Part model, mm, in its own coordinate system. A direction names the side the tool comes from. Coordinates: 2 decimals unless noted, no trailing zeros. Loops run counter-clockwise (first coordinate to the right, second up) from the corner with the lowest first, then second, coordinate; pieces in that order, holes last. Notation, with made-up numbers: (-32.75, -22) - (10.25, -22) arc R23 cw to (10.25, -14) - close; hole circle Ø5 at (14.5, -35). An arc over 180 degrees is marked (long way). Answer as CSV lines item,"result".
Autodesk Inventor part; units mm, degrees
ref_plane "YZ Plane" through (0, 0, 0) normal (1, 0, 0) x (0, 1, 0)
ref_plane "XZ Plane" through (0, 0, 0) normal (0, 1, 0) x (-1, 0, 0)
ref_plane "XY Plane" through (0, 0, 0) normal (0, 0, 1) x (1, 0, 0)
sketch "Sketch1" plane through (0, 0, 0) normal (0, 0, 1) x (1, 0, 0)
  line L0 (-4, -8) -> (16.5, -5)
  line L1 (20, -1.5) -> (20, 1.5)
  line L2 (16.5, 5) -> (-4, 8)
  line L3 (-8, 4) -> (-8, -4)
  line L4 (-4, 8) -> (-8, 4)
  line L5 (-8, -4) -> (-4, -8)
  line L6 (16.5, -5) -> (20, -1.5)
  line L7 (20, 1.5) -> (16.5, 5)
  circle A0 centre (0, 0) radius 2.75
  circle A1 centre (14, 0) radius 2.25
  circle A2 centre (0, 0) radius 5 construction
  circle A3 centre (14, 0) radius 4.5 construction
  point P0 (-8, 0)
  point P1 (20, 0)
  dimension "d9" = 8
  dimension "d10" = 14
  dimension "d11" = 4.5
  dimension "d12" = 5.5
  dimension "d13" = 6
  dimension "d16" = 10
  dimension "d17" = 9
  dimension "d18" = 8
  dimension "d19" = 4
  dimension "d20" = 4
  dimension "d21" = 4
  dimension "d22" = 10
  dimension "d23" = 3
extrude "Extrusion1" add sketch "Sketch1" along normal blind 6.5
sketch "Sketch2" plane through (0, 0, 6.5) normal (0, 0, 1) x (1, 0, 0)
  circle A0 centre (0, 0) radius 2.75
  line L0 (-8, 4) -> (-8, -4)
  line L1 (4.6188, 0) -> (2.3094, -4)
  line L2 (2.3094, -4) -> (-2.3094, -4)
  line L3 (-2.3094, -4) -> (-4.6188, 0)
  line L4 (-4.6188, 0) -> (-2.3094, 4)
  line L5 (-2.3094, 4) -> (2.3094, 4)
  line L6 (2.3094, 4) -> (4.6188, 0)
  dimension "d24" = 8
extrude "Extrusion2" cut sketch "Sketch2" against normal through all
properties part number "y_carriage_nut_holder_a" material "Plywood, Finish"
Q1. Wall check: L1, parallel to Y at x = 1, z = 1.75; L2, parallel to Y at x = 14, z = 2; L3, parallel to Y at x = 6.5, z = 3.25. Give the ranges that are in metal, low to high.
Results:
L1,"y = -7.27 to -4, 4 to 7.27"
L2,"y = -5.37 to -2.25, 2.25 to 5.37"
L3,"y = -6.46 to 6.46"
Q2. Saw through at C-C (x = 14). Give the cut face in (y, z), then the cut area to 3 significant figures.
Results:
outline,"(-5.37, 0) - (-2.25, 0) - (-2.25, 6.5) - (-5.37, 6.5) - close; (2.25, 0) - (5.37, 0) - (5.37, 6.5) - (2.25, 6.5) - close"
area,"40.5 mm^2"
Q3. Which spindle directions (+Z, -Z, +X, -X, +Y, -Y) get a long thin tool onto all of the face, cutting with end or side? Do faces 4 (the face through (3.448, 2.028, 3.296)), 5 (the face through (-6, -6, 3)). Say none if no direction does.
Results:
face 4,"+Z, -Z"
face 5,"+Z, -Z, -X, -Y"
Q4. Saw through at B-B (y = -0.75). Give the cut face in (x, z).
Results:
outline,"(-8, 0) - (-4.19, 0) - (-4.19, 6.5) - (-8, 6.5) - close; (4.19, 0) - (11.88, 0) - (11.88, 6.5) - (4.19, 6.5) - close; (16.12, 0) - (20, 0) - (20, 6.5) - (16.12, 6.5) - close"
Q5. Saw through at D-D (y = 3.25). Give the cut face in (x, z).
Results:
outline,"(-8, 0) - (-2.74, 0) - (-2.74, 6.5) - (-8, 6.5) - close; (2.74, 0) - (18.25, 0) - (18.25, 6.5) - (2.74, 6.5) - close"
Q6. Flat gauge pins, fed straight in: pin 1 (1.5 mm diameter, centred on x = 5.5, z = 4, fed in from +Y); pin 2 (1 mm diameter, centred on x = 12.5, z = 4, fed in from +Y); pin 3 (1.4 mm diameter, centred on x = -0.5, z = 2, fed in from -Y). Where does each tip first touch, or does it go through?
Results:
pin 1,"stops at y = 6.72"
pin 2,"stops at y = 5.66"
pin 3,"stops at y = -7.59"
Q7. Two-plate mould, pull along Y, no slides. Class faces 1 (the face through (6, 0, 6.5)), 2 (the face through (16.146, -0.676, 3.204)), 3 (the face through (-6, 6, 3)): released by +Y, released by -Y, zero draft, split by the parting line, or undercut.
Results:
face 1,"zero draft"
face 2,"undercut"
face 3,"released by +Y"
Q8. Saw through at A-A (z = 3.75). Give the cut face in (x, y).
Results:
outline,"(-8, -4) - (-4, -8) - (16.5, -5) - (20, -1.5) - (20, 1.5) - (16.5, 5) - (-4, 8) - (-8, 4) - close; hole (-4.62, 0) - (-2.31, -4) - (2.31, -4) - (4.62, 0) - (2.31, 4) - (-2.31, 4) - close; hole circle Ø4.5 at (14, 0)"
